Design review of the part shown in the three views and the two pictorial views. Dimensions are in mm from the part's minimum x, y and z. Give positions to 0.01 mm unless a question says otherwise; leave off trailing zeros. Order: outer loops, then holes, each group sorted by start corner. A loop starts at its lowest first (then second) coordinate and runs counter-clockwise, first axis right, second up. Notation, with made-up numbers: (51, 22) -> (104, 22) arc R28 cw to (104, 44) -> close; hole circle Ø7 at (12.5, -18). An arc over 180 degrees is marked (long way). Answer in a Markdown table with one row per item. Add a question column.
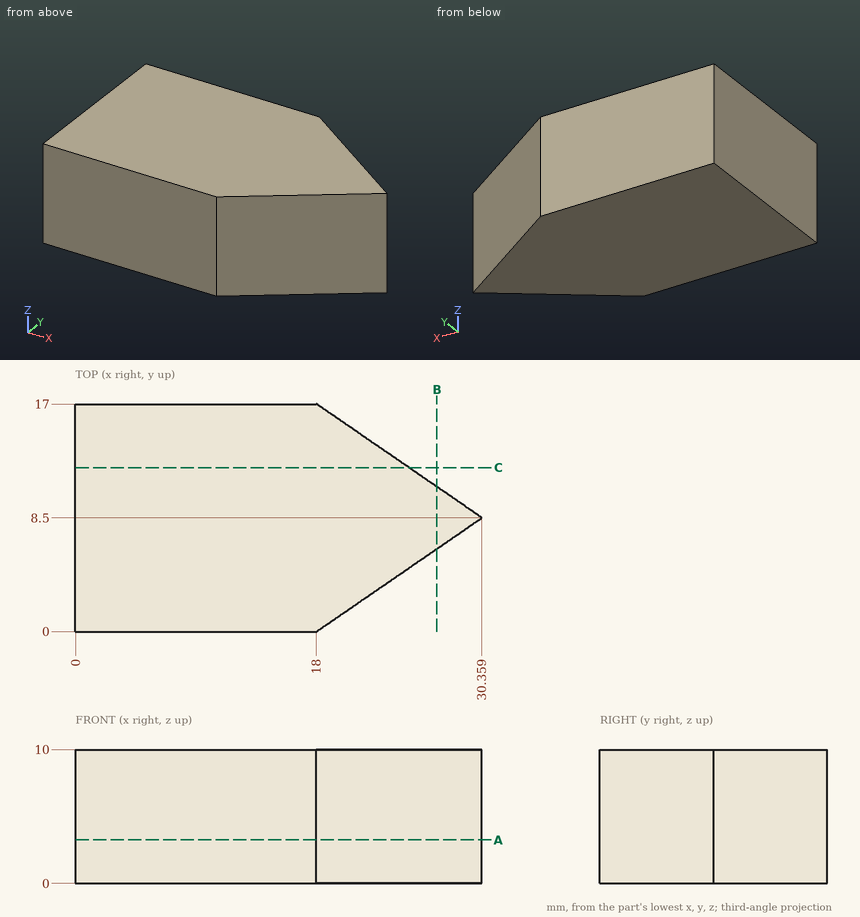
1) Add section B-B, the plane x = 27. Write out the cut boundary in (y, z), and give its area (3 significant figures).
2) Clearance check with a flat-ended pin moving along its axis: P1, Ø3, axis at y = 12.5, z = 7.5, coming from the +X side (1 decimal). State where the tip first meets the part, or that it passes through.
3) For L1, parallel to Y at x = 21, z = 5; L2, parallel to X at y = 14, z = 5.5; L3, parallel to X at y = 10, z = 3.75, list the stretches that pass through material, from the lowest coordinate up.
4) Add section A-A, the plane z = 3.25. Write out the cut boundary in (x, y), and give its area (3 significant figures).
5) Add section C-C, the plane y = 12.25. Write out the cut boundary in (x, z).
Verdict:
| question | item | result |
|---|---|---|
| 1 | outline | (6.19, 0) -> (10.81, 0) -> (10.81, 10) -> (6.19, 10) -> close |
| 1 | area | 46.2 mm2 |
| 2 | P1 | stops at x = 26.7 |
| 3 | L1 | y = 2.06 to 14.94 |
| 3 | L2 | x = 0 to 22.36 |
| 3 | L3 | x = 0 to 28.18 |
| 4 | outline | (0, 0) -> (18, 0) -> (30.36, 8.5) -> (18, 17) -> (0, 17) -> close |
| 4 | area | 411 mm2 |
| 5 | outline | (0, 0) -> (24.91, 0) -> (24.91, 10) -> (0, 10) -> close |
